```python
from build123d import *

# Parameters (mm, degrees)
F0_R     = 2
F0_R_2   = 3
F1_DEPTH = 6.35


with BuildPart() as f1:
    # F0 (on Front) → F1 (new body)
    with BuildSketch(Plane.XZ):
        with BuildLine():
            Line((-6.561359, -10.185191), (-5.030562, 0.706999))
            ThreePointArc((-5.030562, 0.706999), (0.706999, 5.030562), (5.030562, -0.706999))
            Line((5.030562, -0.706999), (3.466391, -11.836654))
            ThreePointArc((3.466391, -11.836654), (3.76555, -12.846599), (4.724031, -13.283404))
            Line((4.724031, -13.283404), (104.14, -13.283404))
            Line((104.14, -13.283404), (104.14, -0.583404))
            Line((104.14, -0.583404), (88.218285, -0.583404))
            ThreePointArc((88.218285, -0.583404), (86.496651, 0.089091), (85.686662, 1.750474))
            ThreePointArc((85.686662, 1.750474), (79.969162, 8.51722), (71.714249, 5.302397))
            ThreePointArc((71.714249, 5.302397), (70.263325, 4.243804), (68.474938, 4.409556))
            Line((68.474938, 4.409556), (40.756691, 17.928649))
            ThreePointArc((40.756691, 17.928649), (39.525036, 19.235869), (39.46594, 21.030948))
            ThreePointArc((39.46594, 21.030948), (36.784215, 29.615632), (27.790551, 29.665466))
            ThreePointArc((27.790551, 29.665466), (26.078277, 29.194234), (24.475846, 29.959843))
            Line((24.475846, 29.959843), (11.334145, 43.568473))
            ThreePointArc((11.334145, 43.568473), (7.839332, 51.063123), (9.69955, 59.120609))
            Line((9.69955, 59.120609), (10.770211, 60.834025))
            Line((10.770211, 60.834025), (0, 67.564))
            Line((0, 67.564), (-16.782521, 40.706351))
            ThreePointArc((-16.782521, 40.706351), (-17.573855, 40.141899), (-18.53254, 40.302328))
            ThreePointArc((-18.53254, 40.302328), (-25.594222, 38.585033), (-23.71271, 31.56532))
            ThreePointArc((-23.71271, 31.56532), (-23.128272, 30.854697), (-23.177073, 29.935909))
            ThreePointArc((-23.177073, 29.935909), (-24.332809, 26.984273), (-25.184893, 23.931106))
            ThreePointArc((-25.184893, 23.931106), (-25.693727, 23.17112), (-26.581209, 22.950068))
            ThreePointArc((-26.581209, 22.950068), (-32.288901, 18.045609), (-26.852685, 12.841859))
            ThreePointArc((-26.852685, 12.841859), (-25.978347, 12.57349), (-25.511038, 11.787288))
            ThreePointArc((-25.511038, 11.787288), (-19.712251, -1.748383), (-8.377773, -11.148912))
            ThreePointArc((-8.377773, -11.148912), (-7.223774, -11.130317), (-6.561359, -10.185191))
        make_face()
        with Locations((-27.210732, 17.909225)):
            Circle(F0_R, mode=Mode.SUBTRACT)
        with BuildLine():
            ThreePointArc((-5.974766, 12.627869), (-13.83499, 13.441854), (-16.746761, 20.788097))
            ThreePointArc((-16.746761, 20.788097), (-11.06787, 32.320826), (0, 38.859624))
            ThreePointArc((0, 38.859624), (6.56969, 38.742325), (12.20146, 35.357395))
            Line((12.20146, 35.357395), (25.602229, 21.480493))
            ThreePointArc((25.602229, 21.480493), (26.624637, 19.42986), (26.285949, 17.16365))
            Line((26.285949, 17.16365), (20.103772, 4.488308))
            ThreePointArc((20.103772, 4.488308), (16.488785, 2.353271), (13.105216, 4.838823))
            ThreePointArc((13.105216, 4.838823), (5.279976, 12.933784), (-5.974766, 12.627869))
        make_face(mode=Mode.SUBTRACT)
        with Locations((32.253298, 23.489035)):
            Circle(F0_R_2, mode=Mode.SUBTRACT)
        with BuildLine():
            ThreePointArc((30.036949, 13.265985), (32.220939, 15.198217), (35.131548, 15.020196))
            Line((35.131548, 15.020196), (62.706484, 1.571001))
            ThreePointArc((62.706484, 1.571001), (64.74864, -2.710467), (61.03629, -5.663404))
            Line((61.03629, -5.663404), (26.901744, -5.663404))
            ThreePointArc((26.901744, -5.663404), (23.67068, -3.872396), (23.477338, -0.18321))
            Line((23.477338, -0.18321), (30.036949, 13.265985))
        make_face(mode=Mode.SUBTRACT)
        with Locations((78.091794, 1.132107)):
            Circle(F0_R_2, mode=Mode.SUBTRACT)
        with Locations((-21.22453, 35.994243)):
            Circle(F0_R, mode=Mode.SUBTRACT)
    extrude(amount=F1_DEPTH)


solid = f1.part
```
Here's how the part is built. I have some questions about the finished solid (model axes, mm). A direction names the side the tool comes from. Round coordinates to 2 decimals unless told otherwise and drop trailing zeros. Order: outer loops, then holes, each group sorted by start corner. A loop starts at its lowest first (then second) coordinate and runs counter-clockwise, first axis right, second up. Notation, with made-up numbers: M 52,-29.75 L 101,-29.75 A23 cw 101,-8.75 Z; hole C 10,85 d6. An arc over 180 degrees is marked long. Answer as CSV lines item,"result".
Item 1: Imagine slicing it at C-C on x = 94. List the corners of the cut face in (y, z) for me, and give its area (3 significant figures).
From the geometry:
outline,"M -6.35,-13.28 L 0,-13.28 L 0,-0.58 L -6.35,-0.58 Z"
area,"80.6 mm2"
Item 2: Imagine slicing it at D-D on z = 51. List the corners of the cut face in (x, y) for me, and give its area (3 significant figures).
From the geometry:
outline,"M -10.35,-6.35 L 7.85,-6.35 L 7.85,0 L -10.35,0 Z"
area,"116 mm2"
Item 3: Imagine slicing it at A-A on z = -8. List the corners of the cut face in (x, y) for me.
From the geometry:
outline,"M -13.5,-6.35 L -6.25,-6.35 L -6.25,0 L -13.5,0 Z; M 4.01,-6.35 L 104.14,-6.35 L 104.14,0 L 4.01,0 Z"
Item 4: We'd pull the mould along X, two halves only. Please class faces 1 (the flat face through (104.14, -3, -7)), 2 (the cylindrical face through (80.097, -3.131, 8.484)), 3 (the flat face through (26, 0, 15)): +X half, -X half, draft (parallel to the pull), parting line (faces both ways), or undercut.
From the geometry:
face 1,"+X half"
face 2,"undercut"
face 3,"draft"
Item 5: For pin 1 (2 mm diameter, centred on y = -4, z = 49.5, fed in from +X); pin 2 (1.5 mm diameter, centred on y = -4.5, z = 7.5, fed in from +X); pin 3 (3 mm diameter, centred on x = 42, z = -2.5, fed in from +Y); pin 4 (4.5 mm diameter, centred on x = -27.21, z = 17.91, fed in from -Y), each with a flat end and sliding along its axis, tell me the tip position at first contact or that it passes through.
From the geometry:
pin 1,"x = 8.38"
pin 2,"x = 83.24"
pin 3,"through"
pin 4,"y = -6.35"
Item 6: Which directions (+Z, -Z, +X, -X, +Y, -Y) give clear straight access to the entire face, cutting with the end or side of a thin tool? Please do faces 4 (the cylindrical face through (-11.19, -3.13, 32.19)), 5 (the cylindrical face through (39.535, -3.131, 19.212)), 6 (the cylindrical face through (-24.319, -3.131, 27.026)).
From the geometry:
face 4,"+Y, -Y"
face 5,"+X, +Y, -Y"
face 6,"-X, +Y, -Y"
Item 7: Please list where these lines run through material, in increasing order: L1, parallel to X at y = -6, z = 4.5; L2, parallel to X at y = -3, z = -2; L3, parallel to Z at x = 9, y = -5. Write a range as [from, to].
From the geometry:
L1,"[-23.34, -2.36], [2.36, 13.25], [20.11, 25.76], [56.7, 68.29], [70.87, 84.93]"
L2,"[-19.52, -5.41], [4.85, 23.09], [64.84, 104.14]"
L3,"[-13.28, 10.68], [37.76, 46.94], [57.84, 61.94]"
Item 8: Imagine slicing it at B-B on x = 18. List the corners of the cut face in (y, z) for me.
From the geometry:
outline,"M -6.35,-13.28 L 0,-13.28 L 0,2.58 L -6.35,2.58 Z; M -6.35,29.35 L 0,29.35 L 0,36.67 L -6.35,36.67 Z"
